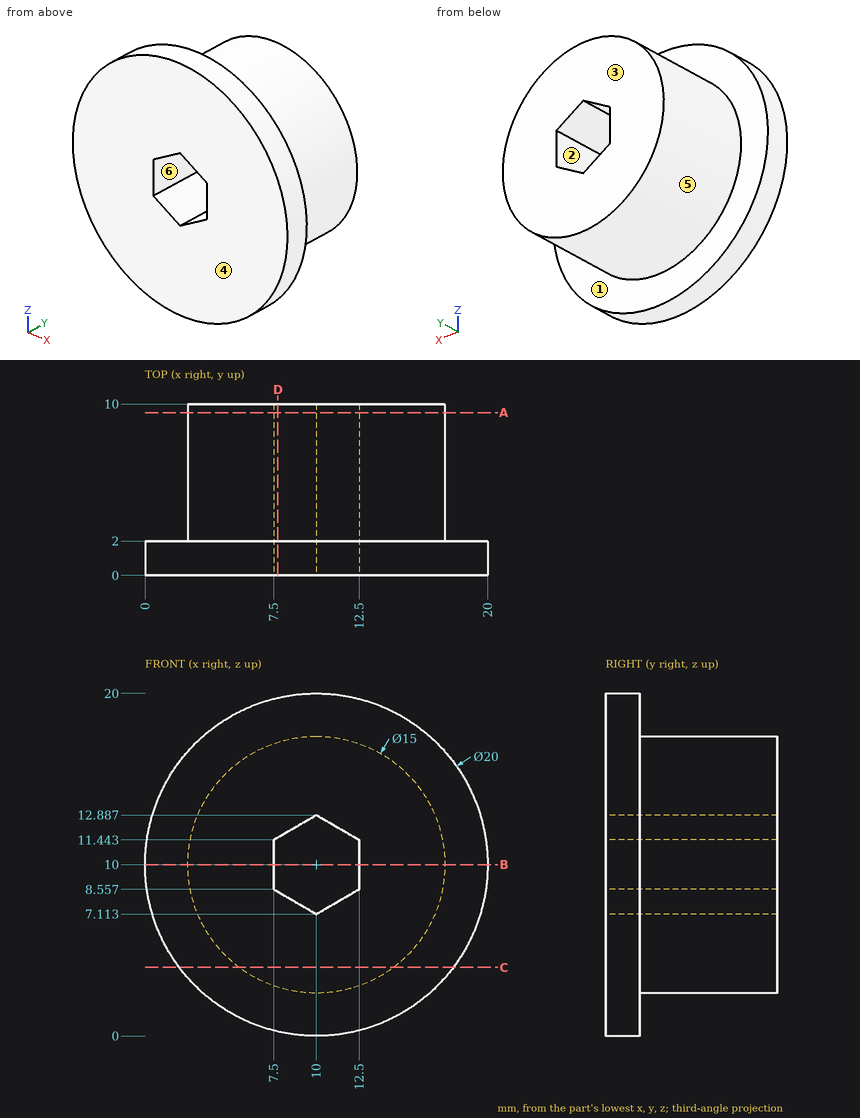
The figure shows three views and two pictorial views of one solid part (mm, origin at its lowest corner). Answer the questions. A direction names the side the tool comes from. Round coordinates to 2 decimals unless told otherwise and drop trailing zeros. Order: outer loops, then holes, each group sorted by start corner. A loop starts at its lowest first (then second) coordinate and runs counter-clockwise, first axis right, second up. Notation, with made-up numbers: (-2.75, 77) -> (37.25, 77) arc R21 ccw to (37.25, 81) -> close; hole circle Ø7 at (66, -38.5). An arc over 180 degrees is marked (long way). One line per item, written item: value.
Item 1: Find section B-B, the plane z = 10. Give the vertices of the cut face in (x, y), then the cut area to 3 significant figures.
Taken from the geometry:
outline: (0, 0) -> (7.5, 0) -> (7.5, 10) -> (2.5, 10) -> (2.5, 2) -> (0, 2) -> close; (12.5, 0) -> (20, 0) -> (20, 2) -> (17.5, 2) -> (17.5, 10) -> (12.5, 10) -> close
area: 110 mm2
Item 2: Straight lines are drawn through the part: L1, parallel to X at y = 9, z = 9.75; L2, parallel to Z at x = 8.5, y = 9.5. For each, find the intervals that lie inside material, in ascending order.
Taken from the geometry:
L1: x = 2.5 to 7.5, 12.5 to 17.5
L2: z = 2.65 to 7.98, 12.02 to 17.35
Item 3: Find section C-C, the plane z = 4. Give the vertices of the cut face in (x, y), then the cut area to 3 significant figures.
Taken from the geometry:
outline: (2, 0) -> (18, 0) -> (18, 2) -> (14.5, 2) -> (14.5, 10) -> (5.5, 10) -> (5.5, 2) -> (2, 2) -> close
area: 104 mm2
Item 4: Given P1, Ø1, axis at y = 4, z = 3, coming from the -X side; P2, Ø1, axis at x = 5, y = 9, coming from the -Z side; P3, Ø3, axis at x = 9, y = 8, coming from the +Z side, each flat-ended and moving along its own axis, determine where each tip first touches the part or whether it passes through.
Taken from the geometry:
P1: stops at x = 6.26
P2: stops at z = 4
P3: stops at z = 17.5
Item 5: For a pull along Z with two mould halves and no side action, classify the marked faces 4, 5 and 6 as released by +Z, released by -Z, zero draft, split by the parting line, or undercut.
Taken from the geometry:
face 4: zero draft
face 5: split by the parting line
face 6: undercut
Item 6: For the marked faces 1, 2 and 3, determine the directions among +Z, -Z, +X, -X, +Y, -Y from which every point of the face is accessible in a straight line to the end or side of a thin tool.
Taken from the geometry:
face 1: +Y
face 2: +Y, -Y
face 3: +Z, -Z, +X, -X, +Y
Item 7: Find section D-D, the plane x = 7.75. Give the vertices of the cut face in (y, z) (1 decimal).
Taken from the geometry:
outline: (0, 0.3) -> (2, 0.3) -> (2, 2.8) -> (10, 2.8) -> (10, 8.4) -> (0, 8.4) -> close; (0, 11.6) -> (10, 11.6) -> (10, 17.2) -> (2, 17.2) -> (2, 19.7) -> (0, 19.7) -> close
Item 8: Find section A-A, the plane y = 9.5. Give the vertices of the cut face in (x, z).
Taken from the geometry:
outline: circle Ø15 at (10, 10); hole (7.5, 8.56) -> (10, 7.11) -> (12.5, 8.56) -> (12.5, 11.44) -> (10, 12.89) -> (7.5, 11.44) -> close
